Geometry check sheet. Reference: the model listing, model coordinates, mm. A direction names the side the tool comes from. Round coordinates to 2 decimals unless told otherwise and drop trailing zeros. Order: outer loops, then holes, each group sorted by start corner. A loop starts at its lowest first (then second) coordinate and runs counter-clockwise, first axis right, second up.
(1) Cross-section at D-D on x = 4. Enter the section's corners in (y, z), and give its area (3 significant figures).
(2) Draft check along Y on faces 3 (the face through (17, -6.35, 6)), 4 (the face through (-1.38, -6.2, 12.52)), 5 (the face through (3, 6, 25.4)). Enter one of: pulls with the +Y half, pulls with the -Y half, needs draft (parallel to the pull), parting line crosses it, or undercut.
(3) Gauge pin test, flat ends, axial feed: P1, Ø4, axis at x = 3.5, z = 14, coming from the -Y side; P2, Ø8, axis at y = -1.5, z = 19, coming from the +X side; P3, Ø13.5, axis at x = 15, z = 8, coming from the +Y side. Record the tip position at first contact, or that the pin passes through.
(4) Set-up check for faces 1 (the face through (20.103, -0.089, 9.569)), 2 (the face through (17, 6.35, 6)): record each of +Z, -Z, +X, -X, +Y, -Y from which the full face is reachable in a straight line by a thin tool's end or side.
(5) Cross-section at C-C on z = 22.5. Enter the section's corners in (x, y), and give its area (3 significant figures).
(6) Cross-section at B-B on y = 0. Enter the section's corners in (x, z).
(7) Thickness scan on L1, parallel to Y at x = 0, z = 19; L2, parallel to Z at x = 15, y = -2.5; L3, parallel to X at y = -1.25, z = 15. Record the ranges inside material, lowest first.
(8) Cross-section at A-A on x = 0. Enter the section's corners in (y, z).
from build123d import *

# Parameters (mm, degrees)
F0_R     = 12.7
F0_R_2   = 6.35
F1_DEPTH = 25.4
F2_W     = 12.7
F2_H     = 12.7
F3_DEPTH = 6.35
F4_SIZE  = 6.35


with BuildPart() as f1:
    # F0 (on Top) → F1 (new body)
    with BuildSketch(Plane.XY):
        Circle(F0_R)
        Circle(F0_R_2, mode=Mode.SUBTRACT)
    extrude(amount=F1_DEPTH)

    # F2 (on Front) → F3 (join, symmetric)
    with BuildSketch(Plane.XZ):
        with Locations((16.972898, 6.35)):
            Rectangle(F2_W, F2_H)
    extrude(amount=F3_DEPTH, both=True)

    # F4
    f4_edges = [f1.edges().sort_by_distance(p)[0] for p in [
        (23.322898, 0, 12.7),
    ]]
    chamfer(f4_edges, length=F4_SIZE)


solid = f1.part
Found:
1. outline: (-12.05, 0) - (-4.93, 0) - (-4.93, 25.4) - (-12.05, 25.4) - close; (4.93, 0) - (12.05, 0) - (12.05, 25.4) - (4.93, 25.4) - close
1. area: 362 mm2
2. face 3: pulls with the -Y half
2. face 4: undercut
2. face 5: needs draft
3. P1: stops at y = -12.61
3. P2: stops at x = 12.7
3. P3: stops at y = 9.66
4. face 1: +Z, +X, +Y, -Y
4. face 2: +Z, -Z, +X, +Y
5. outline: circle Ø25.4 at (0, 0); hole circle Ø12.7 at (0, 0)
5. area: 380 mm2
6. outline: (-12.7, 0) - (-6.35, 0) - (-6.35, 25.4) - (-12.7, 25.4) - close; (6.35, 0) - (23.32, 0) - (23.32, 6.35) - (16.97, 12.7) - (12.7, 12.7) - (12.7, 25.4) - (6.35, 25.4) - close
7. L1: y = -12.7 to -6.35, 6.35 to 12.7
7. L2: z = 0 to 12.7
7. L3: x = -12.64 to -6.23, 6.23 to 12.64
8. outline: (-12.7, 0) - (-6.35, 0) - (-6.35, 25.4) - (-12.7, 25.4) - close; (6.35, 0) - (12.7, 0) - (12.7, 25.4) - (6.35, 25.4) - close
